from build123d import *

# Parameters (mm, degrees)
F1_DEPTH      = 10
F3_ANGLE      = 30
F5_COUNT      = 6
F6_R          = 30
F6_R_2        = 15
F7_DEPTH      = 13
F7_DEPTH_BACK = 4
F8_R          = 15
F9_DEPTH      = 25
F9_DEPTH_BACK = 25


with BuildPart() as f1:
    # F0 (on Top) → F1 (new body)
    with BuildSketch(Plane.XY):
        with BuildLine():
            Line((0, 0), (25.8819045103, 96.5925826289))
            ThreePointArc((25.8819045103, 96.5925826289), (13.052619222, 99.1444861374), (0, 100))
            Line((0, 100), (0, 0))
        make_face()
        with BuildLine():
            Line((0, 0), (0, 100))
            ThreePointArc((0, 100), (-13.052619222, 99.1444861374), (-25.8819045103, 96.5925826289))
            Line((-25.8819045103, 96.5925826289), (0, 0))
        make_face()
    extrude(amount=F1_DEPTH)


with BuildPart() as f1_1:
    # F3: moved
    add(f1.part.rotate(Axis((0, 41.2369845435, 0), (0, -1, 0)), F3_ANGLE))

    # F5: F1 ×6 about axis
    f5_axis = Axis((0, 0, 3.0173412524), (0, 0, -1))


with BuildPart() as f1_2:
    add(f1_1.part)
    for i in range(1, F5_COUNT):
        add(f1_1.part.rotate(f5_axis, i * 360 / F5_COUNT))

    # F6 (on Top) → F7 (join, two sides)
    with BuildSketch(Plane.XY) as f7_sk:
        Circle(F6_R)
        Circle(F6_R_2, mode=Mode.SUBTRACT)
    extrude(amount=F7_DEPTH)
    extrude(f7_sk.sketch, amount=-F7_DEPTH_BACK)

    # F8 (on Top) → F9 (cut, two sides)
    with BuildSketch(Plane.XY) as f9_sk:
        Circle(F8_R)
    extrude(amount=-F9_DEPTH, mode=Mode.SUBTRACT)
    extrude(f9_sk.sketch, amount=F9_DEPTH_BACK, mode=Mode.SUBTRACT)


solid = f1_2.part
CAD build for the part. Positions are in the model's coordinates, mm. A direction names the side the tool comes from. Round coordinates to 2 decimals unless told otherwise and drop trailing zeros. Write each loop counter-clockwise with the first axis right and the second up, starting at its lowest first coordinate (ties: lowest second). Pieces come first, ordered by that corner, then holes. Notation, with made-up numbers: M 0.25,-22 L 30.25,-22 A20 ccw 30.25,-14 Z; hole C -29.5,29.25 d6. An arc over 180 degrees is marked long. Put each result on its own line as item: value. Start each with the question number.
1) Pin check, flat tips, straight feed: pin 1 Ø3 at (x, y) = (77, 49.5) entering from +Z; pin 2 Ø1 at (x, z) = (40, 14.5) entering from -Y; pin 3 Ø1.5 at (x, y) = (17.5, -20) entering from +Z. Stop position of each tip, or through.
2) Pull direction X, two halves, no side cores. Call faces 4 (the flat face through (62.754, -16.599, -4.123)), 5 (the flat face through (-5.31, 72.4, 8.48)), 6 (the flat face through (-65.36, 31.6, 8.48)): pulls with the +X half, pulls with the -X half, needs draft (parallel to the pull), parting line crosses it, or undercut.
3) 3-axis set-ups, long thin cutter, end or side, ignore diameter. For faces 1 (the flat face through (45.75, 46.05, -4.12)), 2 (the flat face through (6, 14, 13)), 3 (the flat face through (-45.75, -46.05, -4.12)): which of +Z, -Z, +X, -X, +Y, -Y reach the whole face in a straight line?
4) Saw through at B-B, the plane y = -57. Count the separate pieces of the cut face and the enclosed holes in it, and give its area (3 significant figures).
5) Drill centre lines: probe 1 along Y at (x, z) = (0, -2.9); probe 2 along Y at (x, z) = (0, 3.5). Where is each one in solid material? Low to high. Write a range as [from, to].
6) Saw through at D-D, the plane x = -44. Write the cut outline in (y, z).
7) Saw through at A-A, the plane x = 65. Write the cut outline in (y, z), and give its area (3 significant figures).
Resolved:
1. pin 1: z = 9.89
1. pin 2: y = -32.09
1. pin 3: z = 13
2. face 4: pulls with the +X half
2. face 5: undercut
2. face 6: pulls with the -X half
3. face 1: -Z, +Y
3. face 2: +Z
3. face 3: -Z, -Y
4. separate pieces: 3
4. enclosed holes: 0
4. area: 789 mm²
5. probe 1: [-30, -15], [15, 30]
5. probe 2: [-99.98, -15], [15, 99.98]
6. outline: M -47.79,0.35 L -41.12,-7.86 L -13.4,6 L -18.49,15 Z; M 8.31,3 L 13.4,-6 L 41.12,7.86 L 34.46,16.07 Z
7. outline: M -60.75,11.61 L -19.79,-8.87 L -14.7,0.13 L -54.08,19.82 Z; M 19.79,8.87 L 60.75,-11.61 L 67.42,-3.4 L 24.88,17.87 Z
7. area: 946 mm²
